Source: CAD feature listing. Evaluate the final solid. Frame: model axes, mm. A direction names the side the tool comes from. Round coordinates to 2 decimals unless told otherwise and drop trailing zeros. Write each loop counter-clockwise with the first axis right and the second up, starting at its lowest first coordinate (ties: lowest second). Pieces come first, ordered by that corner, then holes.
```python
from build123d import *

# Parameters (mm, degrees)
SKETCH2_R           = 30.3149
BOSS_EXTRUDE1_DEPTH = 7.9375


with BuildPart() as part:
    # Sketch1 → Revolve1 (revolve)
    with BuildSketch(Plane.XY):
        Polygon((-56.35625, -44.45), (0, -44.45), (0, -26.2509), (-14.2875, -26.2509), (-14.2875, -30.0863), (-56.35625, -30.3149), align=None)
    revolve(axis=Axis((-56.35625, 0, 0), (1, 0, 0)))

    # Sketch2 → Boss-Extrude1 (add)
    with BuildSketch(Plane.ZY.offset(56.35625)):
        Polygon((0, 53.159526036), (-46.0375, 26.579763018), (-46.0375, -26.579763018), (0, -53.159526036), (46.0375, -26.579763018), (46.0375, 26.579763018), align=None)
        Circle(SKETCH2_R, mode=Mode.SUBTRACT)
    extrude(amount=-BOSS_EXTRUDE1_DEPTH)


solid = part.part
```
Q1. Section query A-A, the plane x = -4. Output: boundary loops of the cut face in (y, z).
Q2. Section query C-C, the plane x = -45. Output: boundary loops of the cut face in (y, z), and give its area (3 significant figures).
Q3. Set-up query: faces 5 (the face through (-23.87, -42.397, -13.352)), 6 (the face through (-35.616, 6.547, 29.484)), 7 (the face through (-52.443, 40.056, -22.696)). Return all of +Z, -Z, +X, -X, +Y, -Y with unobstructed straight access to the full face (end or side cutting, diameter ignored); none if empty.
Q4. Mould query, pull axis Z, two halves, no side actions, for faces 1 (the face through (-52, 0, -46.038)), 2 (the face through (-7.244, 3.417, -26.028)), 3 (the face through (-52.443, 39.684, 23.341)), 4 (the face through (-14.288, -9, -25)). Classes: pulls with the +Z half, pulls with the -Z half, needs draft (parallel to the pull), parting line crosses it, or undercut.
Q5. Pin query (flat end, axial travel): P1, Ø1, axis at x = -15.5, y = 26, coming from the -Z side; P2, Ø6, axis at x = -22.5, y = -11.5, coming from the +Z side; P3, Ø2, axis at x = -27, z = 22, coming from the -Y side. Return the tip coordinate at first contact, or that it passes through.
Q6. Line query: line 1 (Z direction, x = -8, y = 0); line 2 (Z direction, x = -36, y = 4). Output: solid intervals per line, ascending.
Q7. Section query B-B, the plane y = 35.5. Output: boundary loops of the cut face in (x, z), and give its area (3 significant figures).
Filled in:
1. outline: circle Ø88.9 at (0, 0); hole circle Ø52.5 at (0, 0)
2. outline: circle Ø88.9 at (0, 0); hole circle Ø60.51 at (0, 0)
2. area: 3,330 mm2
3. face 5: +X
3. face 6: -X
3. face 7: -Z, +X, -X, +Y
4. face 1: pulls with the -Z half
4. face 2: undercut
4. face 3: pulls with the +Z half
4. face 4: undercut
5. P1: stops at z = -36.41
5. P2: stops at z = 43.63
5. P3: stops at y = -39.18
6. line 1: z = -44.45 to -26.25, 26.25 to 44.45
6. line 2: z = -44.27 to -29.94, 29.94 to 44.27
7. outline: (-56.36, -30.59) - (-48.42, -30.59) - (-48.42, -26.75) - (0, -26.75) - (0, 26.75) - (-48.42, 26.75) - (-48.42, 30.59) - (-56.36, 30.59) - close
7. area: 3,080 mm2
